from build123d import *

# Parameters (mm, degrees)
SKETCH1_R           = 16
SKETCH1_R_2         = 9
SKETCH1_R_3         = 7.5
BOSS_EXTRUDE1_DEPTH = 27.5
SKETCH1_3_R         = 9
SKETCH1_3_R_2       = 7.5
BOSS_EXTRUDE2_DEPTH = 2
SKETCH3_R           = 1.5
CUT_EXTRUDE1_DEPTH  = 47
BOSS_EXTRUDE5_START = -27.5
SKETCH1_5_R         = 9
SKETCH1_5_R_2       = 7.5
BOSS_EXTRUDE5_DEPTH = 2
SCALE1_SCALE        = 1.667


with BuildPart() as part:
    # Sketch1 → Boss-Extrude1 (new body)
    with BuildSketch(Plane.XY):
        Circle(SKETCH1_R)
        Circle(SKETCH1_R_2, mode=Mode.SUBTRACT)
        Circle(SKETCH1_R_2)
        Circle(SKETCH1_R_3, mode=Mode.SUBTRACT)
    extrude(amount=-BOSS_EXTRUDE1_DEPTH)

    # Sketch1<3> → Boss-Extrude2 (add)
    with BuildSketch(Plane.XY):
        Circle(SKETCH1_3_R)
        Circle(SKETCH1_3_R_2, mode=Mode.SUBTRACT)
    extrude(amount=BOSS_EXTRUDE2_DEPTH)

    # Sketch3 → Cut-Extrude1 (cut)
    with BuildSketch(Plane.XY):
        with Locations((-8.485281374, 8.485281374)):
            Circle(SKETCH3_R)
        with Locations((8.485281374, 8.485281374)):
            Circle(SKETCH3_R)
        with Locations((8.485281374, -8.485281374)):
            Circle(SKETCH3_R)
        with Locations((-8.485281374, -8.485281374)):
            Circle(SKETCH3_R)
    extrude(amount=-CUT_EXTRUDE1_DEPTH, mode=Mode.SUBTRACT)

    # Sketch1<5> → Boss-Extrude5 (add)
    with BuildSketch(Plane.XY.offset(BOSS_EXTRUDE5_START)):
        Circle(SKETCH1_5_R)
        Circle(SKETCH1_5_R_2, mode=Mode.SUBTRACT)
    extrude(amount=-BOSS_EXTRUDE5_DEPTH)


with BuildPart() as part_1:
    # Scale1: scaled about (0, 0, -13.75)
    add(part.part.scale(SCALE1_SCALE).moved(Location((0, 0, 9.17125))))


solid = part_1.part
For this review, take the finished solid that the model builds, in its own axes (mm). A direction names the side the tool comes from. Give positions to 0.01 mm unless a question says otherwise; leave off trailing zeros. Order: outer loops, then holes, each group sorted by start corner. A loop starts at its lowest first (then second) coordinate and runs counter-clockwise, first axis right, second up. Notation, with made-up numbers: M 84.5,35.5 L 125.5,35.5 A28 ccw 125.5,67.5 Z; hole C 89,72.5 d3. An arc over 180 degrees is marked long. Answer in a Markdown table with one row per item. Add a question column.
(1) Mouldability with a two-part tool opening along Y and no side actions: class faces 1 (the face through (-3.4, 12.3, 12.505)), 2 (the face through (-14.687, 11.704, -13.429)), 3 (the face through (-11.906, -9.129, -38.315)) as +Y half, -Y half, draft (parallel to the pull), parting line (faces both ways), or undercut.
(2) For faces 4 (the face through (16.455, -15.103, -13.429)), 5 (the face through (11, -11, -36.671)), 6 (the face through (11, -11, 9.171)), list the 3-axis set-ups (+Z, -Z, +X, -X, +Y, -Y) from which the entire face can be reached by the end or side of a thin tool; tool diameter is ignored.
(3) Consider section C-C on z = -1.5. State the section outline as (x, y) points (1 decimal), and give its area (3 significant figures).
(4) Consider section D-D on x = 22. State the section outline as (y, z) points.
(5) Wall thickness on probe 1 along X at (y, z) = (14, -24.5); probe 2 along Y at (x, z) = (0, -13): over which ranges is each line inside the solid? List them lowest first. Write a range as [from, to].
(6) Consider section A-A on y = 0. State the section outline as (x, z) points.
(7) For pin 1 (5 mm diameter, centred on x = -5.5, z = -2, fed in from -Y); pin 2 (5 mm diameter, centred on x = 13.5, y = 19.5, fed in from +Z); pin 3 (12 mm diameter, centred on y = -13, z = -11, fed in from -X), all flat-tipped, find the tip position at first contact; note any pin that passes through.
Evaluation:
| question | item | result |
|---|---|---|
| 1 | face 1 | draft |
| 1 | face 2 | undercut |
| 1 | face 3 | parting line |
| 2 | face 4 | +Z, -Z |
| 2 | face 5 | -Z |
| 2 | face 6 | +Z |
| 3 | outline | C 0,0 d53.3; hole C -14.1,-14.1 d5; hole C -14.1,14.1 d5; hole C 0,0 d25; hole C 14.1,-14.1 d5; hole C 14.1,14.1 d5 |
| 3 | area | 1,670 mm^2 |
| 4 | outline | M -15.08,-36.67 L 15.08,-36.67 L 15.08,9.17 L -15.08,9.17 Z |
| 5 | probe 1 | x = [-22.7, -16.64], [-11.65, 11.65], [16.64, 22.7] |
| 5 | probe 2 | y = [-26.67, -12.5], [12.5, 26.67] |
| 6 | outline | M -26.67,-36.67 L -15,-36.67 L -15,-40.01 L -12.5,-40.01 L -12.5,12.51 L -15,12.51 L -15,9.17 L -26.67,9.17 Z; M 12.5,-40.01 L 15,-40.01 L 15,-36.67 L 26.67,-36.67 L 26.67,9.17 L 15,9.17 L 15,12.51 L 12.5,12.51 Z |
| 7 | pin 1 | stops at y = -26.5 |
| 7 | pin 2 | stops at z = 9.17 |
| 7 | pin 3 | stops at x = -25.74 |
